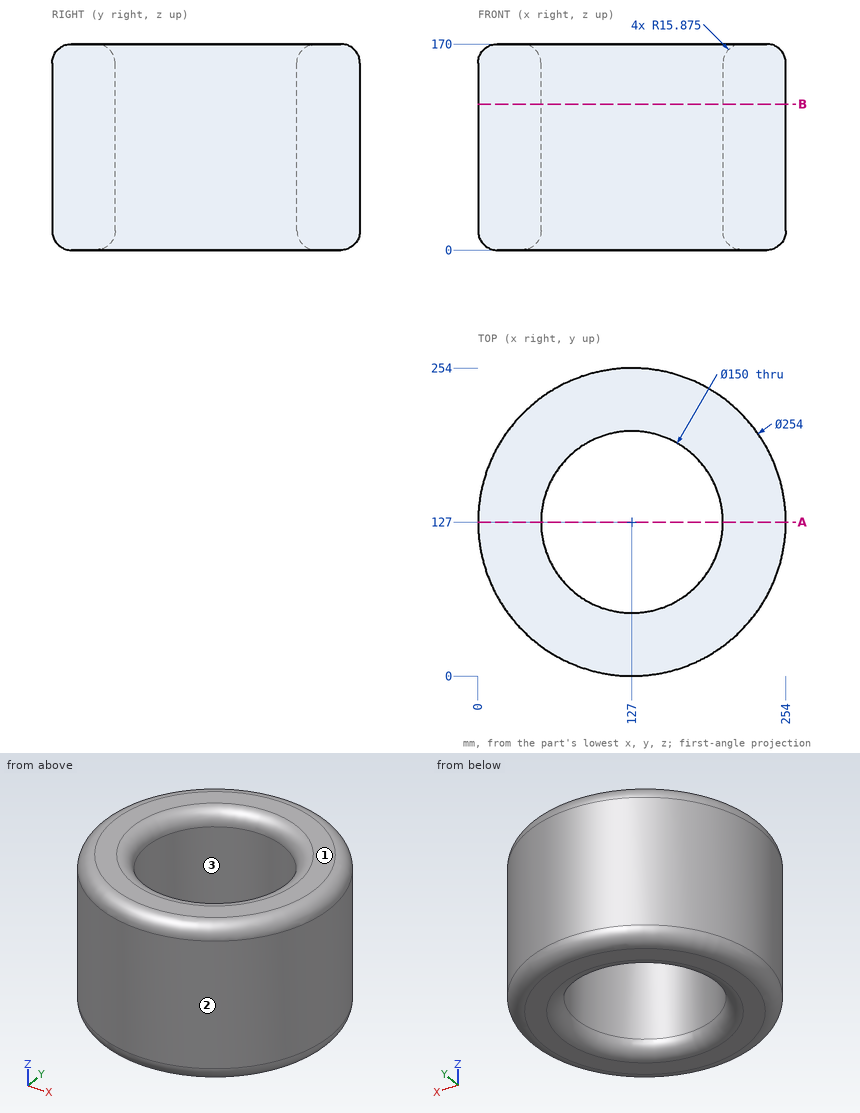
Geometry check sheet. Reference: drawing and pictorial views, mm from the part's lowest x, y, z. Round coordinates to 2 decimals unless told otherwise and drop trailing zeros. Loops run counter-clockwise (first coordinate to the right, second up) from the corner with the lowest first, then second, coordinate; pieces in that order, holes last. Notation, with made-up numbers: (-6, 22.5) -> (36, 22.5) arc R24 ccw to (36, 42.5) -> close; hole circle Ø10 at (-36, 34). An arc over 180 degrees is marked (long way). Use a Markdown table: item, result.
(1) Mould release check, pull along Y, two halves, no side actions. Record for the marked faces 1, 2 and 3: released by +Y, released by -Y, zero draft, split by the parting line, or undercut.
Calculated:
| item | result |
|---|---|
| face 1 | zero draft |
| face 2 | split by the parting line |
| face 3 | undercut |
(2) Sectioned sample at B-B (z = 120.5). Enter the section's corners in (x, y), then the cut area to 3 significant figures.
Calculated:
| item | result |
|---|---|
| outline | circle Ø254 at (127, 127); hole circle Ø150 at (127, 127) |
| area | 33,000 mm² |
(3) Go/stop test with flat-tipped pins: P1, Ø2, axis at x = 148, y = 53, coming from the +Z side; P2, Ø10, axis at x = 108.5, z = 129, coming from the -Y side; P3, Ø12, axis at x = 204, y = 228, coming from the +Z side. Record where each tip stops, or that it passes through.
Calculated:
| item | result |
|---|---|
| P1 | z = 163.3 |
| P2 | y = 0.72 |
| P3 | z = 166.55 |
(4) Scan lines: probe 1 along Y at (x, z) = (127, 66); probe 2 along Y at (x, z) = (130, 143.5); probe 3 along X at (y, z) = (111, 137.5). Record each from-to range of solid material in increasing order.
Calculated:
| item | result |
|---|---|
| probe 1 | 0 to 52, 202 to 254 |
| probe 2 | 0.04 to 52.06, 201.94 to 253.96 |
| probe 3 | 1.01 to 53.73, 200.27 to 252.99 |
(5) Sectioned sample at A-A (y = 127). Enter the section's corners in (x, z) (3 decimals), then the cut area to 3 significant figures.
Calculated:
| item | result |
|---|---|
| outline | (0, 15.875) arc R15.875 ccw to (15.875, 0) -> (36.125, 0) arc R15.875 ccw to (52, 15.875) -> (52, 154.125) arc R15.875 ccw to (36.125, 170) -> (15.875, 170) arc R15.875 ccw to (0, 154.125) -> close; (202, 15.875) arc R15.875 ccw to (217.875, 0) -> (238.125, 0) arc R15.875 ccw to (254, 15.875) -> (254, 154.125) arc R15.875 ccw to (238.125, 170) -> (217.875, 170) arc R15.875 ccw to (202, 154.125) -> close |
| area | 17,200 mm² |
